Read the model definition and answer for the solid it produces. Units are mm, in the model's axes. Give positions to 0.01 mm unless a question says otherwise; leave off trailing zeros. Write each loop counter-clockwise with the first axis right and the second up, starting at its lowest first coordinate (ties: lowest second). Pieces come first, ordered by that corner, then holes. Notation, with made-up numbers: M 5,62 L 11,62 A17 cw 11,83 Z; hole C 24.5,-33 d7. An arc over 180 degrees is marked long. Answer as CSV lines item,"result". Start each with the question number.
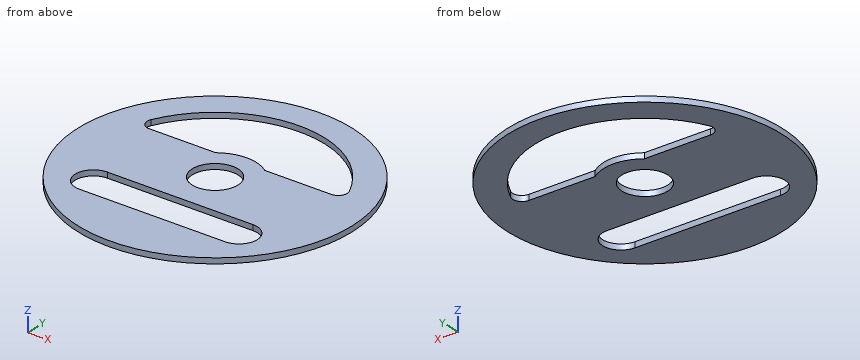
```python
from build123d import *

# Parameters (mm, degrees)
SKETCH1_R           = 75
SKETCH1_R_2         = 12.5
BOSS_EXTRUDE1_DEPTH = 3


with BuildPart() as part:
    # Sketch1 → Boss-Extrude1 (new body)
    with BuildSketch(Plane.XY):
        Circle(SKETCH1_R)
        Circle(SKETCH1_R_2, mode=Mode.SUBTRACT)
        with BuildLine():
            Line((-40, -25), (40, -25))
            ThreePointArc((40, -25), (50, -35), (40, -45))
            Line((40, -45), (-40, -45))
            ThreePointArc((-40, -45), (-50, -35), (-40, -25))
        make_face(mode=Mode.SUBTRACT)
        with BuildLine():
            Line((-49.959983987, 18), (-13.5, 18))
            ThreePointArc((-13.5, 18), (0, 22.5), (13.5, 18))
            Line((13.5, 18), (49.959983987, 18))
            ThreePointArc((49.959983987, 18), (54.170360779, 20.30320055), (54.501800713, 25.090909091))
            ThreePointArc((54.501800713, 25.090909091), (0, 60), (-54.501800713, 25.090909091))
            ThreePointArc((-54.501800713, 25.090909091), (-54.170360779, 20.30320055), (-49.959983987, 18))
        make_face(mode=Mode.SUBTRACT)
    extrude(amount=BOSS_EXTRUDE1_DEPTH)


solid = part.part
```
1. Find section C-C on x = 30. Determine the outline of the cut face in (y, z).
2. Find section B-B on z = 0.75. Determine the outline of the cut face in (x, y).
3. Given pin 1 (1.5 mm diameter, centred on x = -25, z = 1, fed in from +Y); pin 2 (1.5 mm diameter, centred on x = -2.5, z = 1, fed in from +Y), each flat-ended and moving along its own axis, determine where each tip first touches the part or whether it passes through.
4. Find section D-D on y = -35. Determine the outline of the cut face in (x, z).
5. Find section A-A on x = 0. Determine the outline of the cut face in (y, z), then the cut area to 4 significant figures.
6. Find the intervals of material crossed by line 1 (Y direction, x = 0, z = 2); line 2 (Y direction, x = 38.5, z = 0.7); line 3 (Y direction, x = -28, z = 2.1), in increasing order. Write a range as [from, to].
Computed:
1,outline,"M -68.74,0 L -45,0 L -45,3 L -68.74,3 Z; M -25,0 L 18,0 L 18,3 L -25,3 Z; M 51.96,0 L 68.74,0 L 68.74,3 L 51.96,3 Z"
2,outline,"C 0,0 d150; hole M -54.5,25.09 A5 ccw -49.96,18 L -13.5,18 A22.5 cw 13.5,18 L 49.96,18 A5 ccw 54.5,25.09 A60 ccw Z; hole M -40,-45 L 40,-45 A10 ccw 40,-25 L -40,-25 A10 ccw Z; hole C 0,0 d25"
3,pin 1,"stops at y = 70.97"
3,pin 2,"stops at y = 74.98"
4,outline,"M -66.33,0 L -50,0 L -50,3 L -66.33,3 Z; M 50,0 L 66.33,0 L 66.33,3 L 50,3 Z"
5,outline,"M -75,0 L -45,0 L -45,3 L -75,3 Z; M -25,0 L -12.5,0 L -12.5,3 L -25,3 Z; M 12.5,0 L 22.5,0 L 22.5,3 L 12.5,3 Z; M 60,0 L 75,0 L 75,3 L 60,3 Z"
5,area,"202.5 mm^2"
6,line 1,"y = [-75, -45], [-25, -12.5], [12.5, 22.5], [60, 75]"
6,line 2,"y = [-64.36, -45], [-25, 18], [46.02, 64.36]"
6,line 3,"y = [-69.58, -45], [-25, 18], [53.07, 69.58]"
